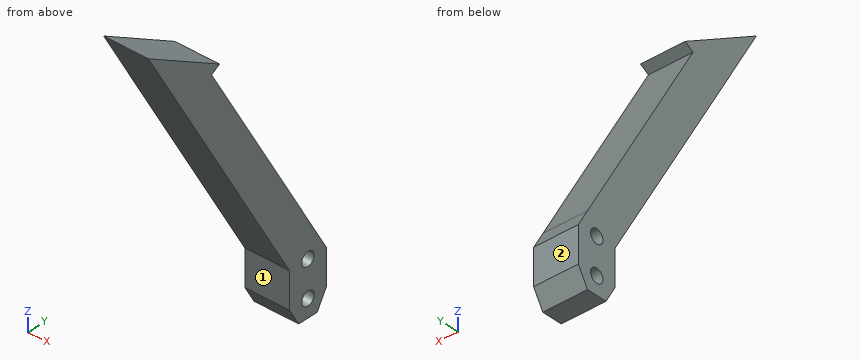
Autodesk Inventor part; units mm, degrees
ref_plane "YZ Plane" through (0, 0, 0) normal (1, 0, 0) x (0, 1, 0)
ref_plane "XZ Plane" through (0, 0, 0) normal (0, 1, 0) x (-1, 0, 0)
ref_plane "XY Plane" through (0, 0, 0) normal (0, 0, 1) x (1, 0, 0)
sketch "Sketch1" plane through (0, 0, 0) normal (1, 0, 0) x (0, 1, 0)
  line L0 (2.3094, 8) -> (-2.3094, 8)
  line L1 (-2.3094, 8) -> (-2.3094, -8)
  line L2 (-2.3094, -8) -> (2.3094, -8)
  line L3 (2.3094, -8) -> (2.3094, 8)
  line L4 (2.3094, 8) -> (-2.3094, -8) construction
  line L5 (-2.3094, 8) -> (2.3094, -8) construction
  line L6 (2.3094, 8) -> (-24.153, 53.8342)
  line L7 (2.3094, -8) -> (-2.3094, -8)
  line L8 (-2.3094, -8) -> (-4.6188, -4)
  line L9 (-4.6188, -4) -> (-2.3094, 0)
  line L10 (-2.3094, 0) -> (2.3094, 0)
  line L11 (2.3094, 0) -> (4.6188, -4)
  line L12 (4.6188, -4) -> (2.3094, -8)
  line L13 (0, -22.6597) -> (0, 79.958)
  line L14 (2.3094, 8) -> (4.6188, 4)
  line L15 (4.6188, 4) -> (2.3094, 0)
  line L16 (2.3094, 0) -> (-2.3094, 0)
  line L17 (-2.3094, 0) -> (-4.6188, 4)
  line L18 (-4.6188, 4) -> (-2.3094, 8)
  line L19 (-2.3094, 8) -> (2.3094, 8)
  line L20 (4.6188, 4) -> (4.6188, -4)
  line L21 (-4.6188, 4) -> (-4.6188, -4)
  circle A0 centre (0, -4) radius 1.55
  circle A1 centre (0, 4) radius 1.55
  line L22 (2.3094, 8) -> (2.3094, 5.0078)
  line L23 (-40.0094, 65.2983) -> (-22.153, 54.9889)
  line L24 (-22.153, 54.9889) -> (-24.153, 53.8342)
  line L25 (-4.6188, 4) -> (-40.0094, 65.2983)
  point P0 (0, 0)
  point P1 (2.3094, 8)
  point P2 (-3.4641, 6)
  point P3 (0, 8)
  point P4 (0, 12)
  dimension "d3" = 4.6188
  dimension "d4" = 16
  dimension "d15" = 8
  dimension "d16" = 8
  dimension "d18" = 3.1
  dimension "d19" = 3.1
  dimension "d20" = 4.6188
  dimension "d23" = 2
  dimension "d24" = 40.0094
  dimension "d25" = 60
  dimension "d26" = 30
  dimension "d27" = 73.2983
extrude "Extrusion2" add sketch "Sketch1" along normal blind 10 contours L3 L10 L13 A1 L0 | L14 L15 L3 | L0 L13 L6 | L13 A1 L10 L1 L0 | L0 L18 L25 L23 L24 L6 L13 | L20 L11 L15 | L1 L17 L18 | L11 L12 L3 | L3 L2 L13 A0 L10 | L10 L13 A0 L2 L1 | L1 L8 L9 | L9 L21 L17
equation "\"d3\" = FlipperArmThickness"
equation "\"d4\" = 2 * M3ScrewInsertBrim"
equation "\"d15\" = M3ScrewInsertBrim"
equation "\"d16\" = M3ScrewInsertBrim"
equation "\"d18\" = M3ScrewDia"
equation "\"d19\" = M3ScrewDia"
equation "\"d23\" = FlipperSpikeTipOffset"
equation "\"d24\" = FlipperSpikeDrop"
equation "\"d25\" = FlipperSpikeTipAngle"
equation "\"d26\" = FlipperSpikeAngle"
equation "\"d32\" = FlipperSpikeWidth"
equation "\"FlipperSpikeReach\" = d27 - 0.433013 * BodyHeight"
equation "\"FlipperSpikeTipAngle\" = 60deg"
equation "\"FlipperSpikeTipOffset\" = 2"
properties part number "HexFlipperSpike" material "H TPU"
Input: part model. Units: mm. Frame: model coordinates. Face numbers are marked on the shaded views. A direction names the side the tool comes from. Round coordinates to 2 decimals unless told otherwise and drop trailing zeros. Loops run counter-clockwise (first coordinate to the right, second up) from the corner with the lowest first, then second, coordinate; pieces in that order, holes last. Notation, with made-up numbers: (-40, 54.5) -> (-19, 54.5) arc R24 ccw to (-19, 85.5) -> close; hole circle Ø10 at (75, 80.25). An arc over 180 degrees is marked (long way). Use one line per item in the form item = value. Start each with the question number.
Item 1: Section query B-B on z = 21.5. Return the cut outline in (x, y), then the cut area to 3 significant figures.
Item 2: Section query A-A on y = 0. Return the cut outline in (x, z), then the cut area to 3 significant figures.
Item 3: Contact query for flat-ended pins moving along their axis: pin 1 Ø4 at (x, z) = (1.5, 30) entering from +Y; pin 2 Ø6 at (x, y) = (5, -28.5) entering from -Z; pin 3 Ø3 at (x, y) = (2, -26) entering from -Z; pin 4 Ø2.5 at (y, z) = (0, 4) entering from -X. Output: stop coordinate, or through.
Item 4: Section query C-C on y = -27. Return the cut outline in (x, z), then the cut area to 3 significant figures.
Item 5: Set-up query: the marked faces 1 and 2. Return all of +Z, -Z, +X, -X, +Y, -Y with unobstructed straight access to the full face (end or side cutting, diameter ignored); none if empty.
Item 6: Material intervals for L1, parallel to Y at x = 4, z = -4; L2, parallel to Z at x = 6.5, y = 0; L3, parallel to Y at x = 1, z = -3, sorted ascending. Write a range as from..to.
Ans:
q1.outline = (0, -14.72) -> (10, -14.72) -> (10, -5.48) -> (0, -5.48) -> close
q1.area = 92.4 mm^2
q2.outline = (0, -8) -> (10, -8) -> (10, -5.55) -> (0, -5.55) -> close; (0, -2.45) -> (10, -2.45) -> (10, 2.45) -> (0, 2.45) -> close; (0, 5.55) -> (10, 5.55) -> (10, 12) -> (0, 12) -> close
q2.area = 138 mm^2
q3.pin_1 = -9.24
q3.pin_2 = 40.17
q3.pin_3 = 38.44
q3.pin_4 = through
q4.outline = (0, 42.77) -> (10, 42.77) -> (10, 57.79) -> (0, 57.79) -> close
q4.area = 150 mm^2
q5.face_1 = -Z, +X, -X, -Y
q5.face_2 = +Z, -Z, +X, -X, +Y
q6.L1 = -4.62..-1.55, 1.55..4.62
q6.L2 = -8..-5.55, -2.45..2.45, 5.55..12
q6.L3 = -4.62..-1.18, 1.18..4.62
